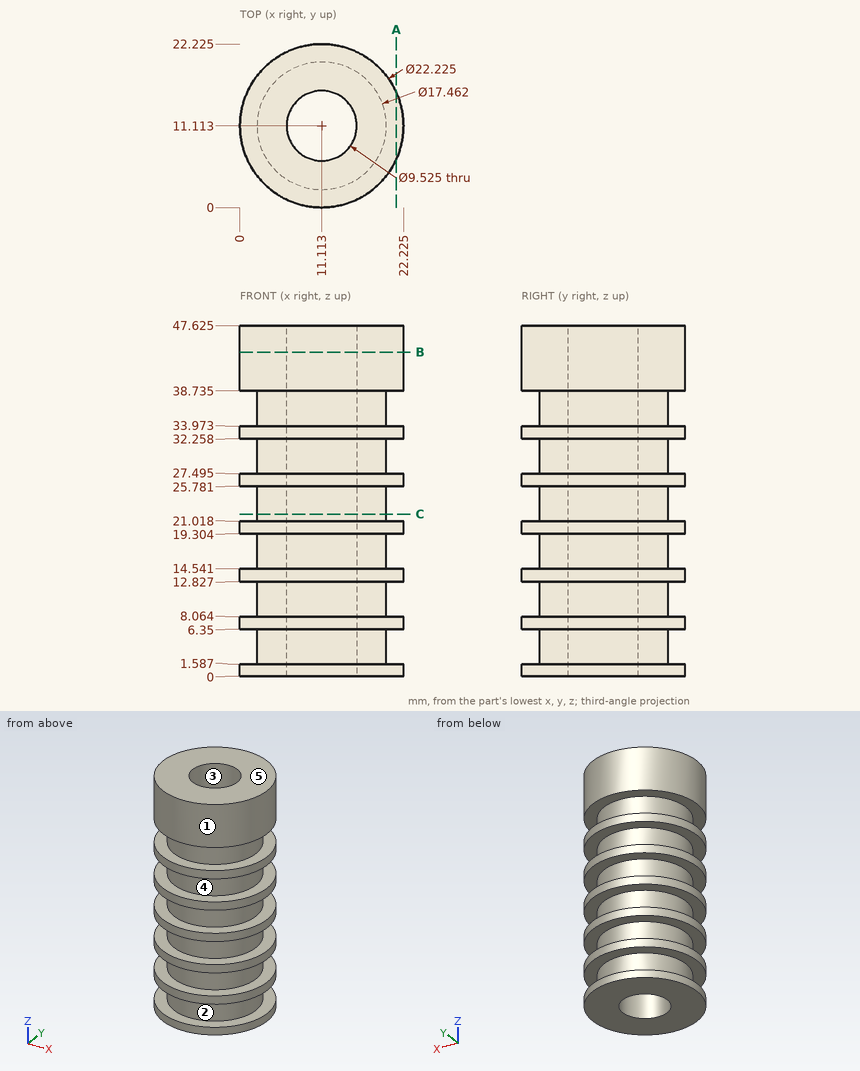
Source: three-view drawing plus pictorial views. Frame: mm from the lowest corner of the part. A direction names the side the tool comes from. Coordinates: 2 decimals unless noted, no trailing zeros. Order: outer loops, then holes, each group sorted by start corner. A loop starts at its lowest first (then second) coordinate and runs counter-clockwise, first axis right, second up. Notation, with made-up numbers: M 44.25,27 L 89.25,27 A11 cw 89.25,36 Z; hole C 21,8.5 d2. An arc over 180 degrees is marked long. Answer in a Markdown table with one row per item.
(1) Section query C-C, the plane z = 22. Output: boundary loops of the cut face in (x, y) (1 decimal).
Numbers:
| item | result |
|---|---|
| outline | C 11.1,11.1 d17.5; hole C 11.1,11.1 d9.5 |
(2) Material intervals for line 1 (X direction, y = 11, z = 4); line 2 (Y direction, x = 9.25, z = 18) (1 decimal); line 3 (X direction, y = 13.5, z = 32) (1 decimal), sorted ascending. Write a range as [from, to].
Numbers:
| item | result |
|---|---|
| line 1 | x = [2.38, 6.35], [15.87, 19.84] |
| line 2 | y = [2.6, 6.7], [15.5, 19.6] |
| line 3 | x = [2.7, 7], [15.2, 19.5] |
(3) Access query for the marked faces 1 and 2. Directions: +Z, -Z, +X, -X, +Y, -Y. A direction counts if a zero-diameter tool reaches every point of the face in a straight line with its end or side. Return the directions, or none.
Numbers:
| item | result |
|---|---|
| face 1 | +Z, -Z |
| face 2 | none |
(4) Draft query along X for the marked faces 3, 4 and 5. Return one class per face: pulls with the +X half, pulls with the -X half, needs draft (parallel to the pull), parting line crosses it, or undercut.
Numbers:
| item | result |
|---|---|
| face 3 | undercut |
| face 4 | parting line crosses it |
| face 5 | needs draft |
(5) Section query B-B, the plane z = 44. Output: boundary loops of the cut face in (x, y) (1 decimal), plus the area to 3 significant figures.
Numbers:
| item | result |
|---|---|
| outline | C 11.1,11.1 d22.2; hole C 11.1,11.1 d9.5 |
| area | 317 mm^2 |
(6) Section query A-A, the plane x = 21.25. Give the number of separate pieces and of enclosed holes in the cut face.
Numbers:
| item | result |
|---|---|
| separate pieces | 7 |
| enclosed holes | 0 |
(7) Contact query for flat-ended pins moving along their axis: pin 1 Ø1 at (x, z) = (18.5, 10.5) entering from +Y; pin 2 Ø1.5 at (y, z) = (3.5, 34.5) entering from -X (1 decimal). Output: stop coordinate, or through.
Numbers:
| item | result |
|---|---|
| pin 1 | stops at y = 16.48 |
| pin 2 | stops at x = 2.5 |
